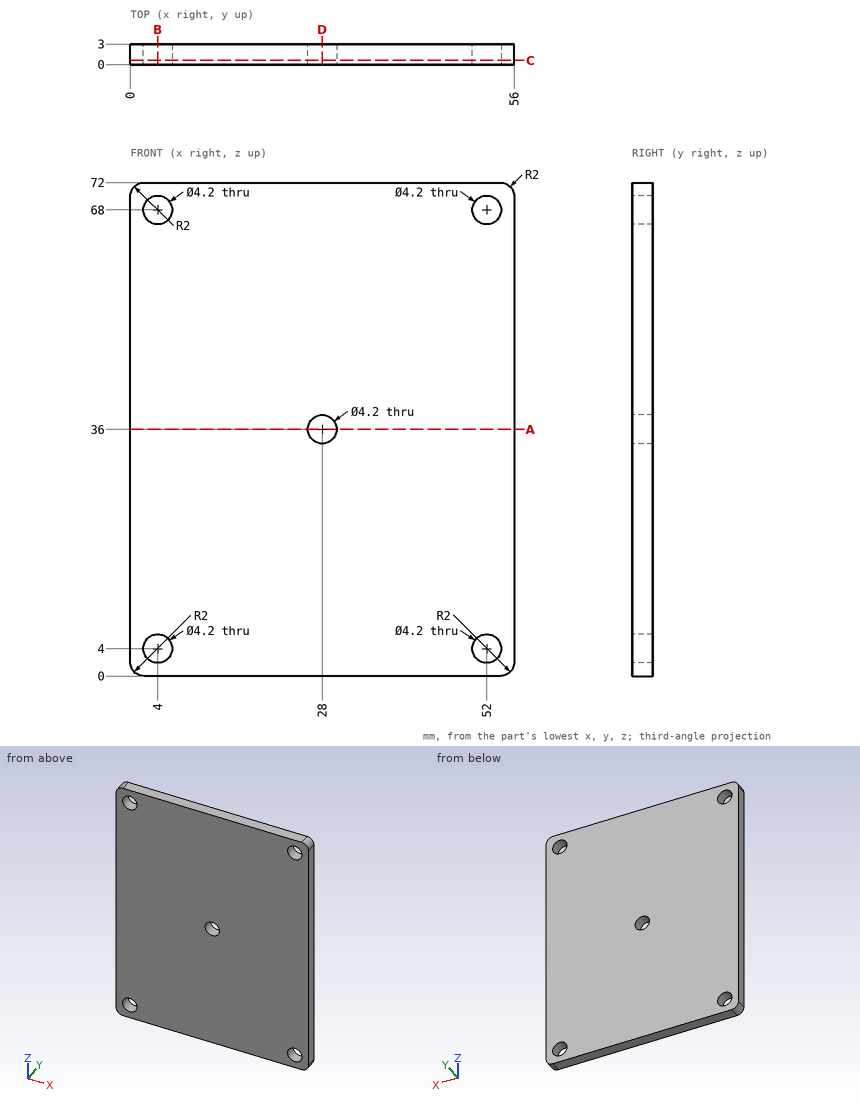
Drawing for the job (mm, zero at the part's lowest x, y, z). Round coordinates to 2 decimals unless told otherwise and drop trailing zeros. Write each loop counter-clockwise with the first axis right and the second up, starting at its lowest first coordinate (ties: lowest second). Pieces come first, ordered by that corner, then holes. Notation, with made-up numbers: (77.5, 45.25) - (112.5, 45.25) arc R35 cw to (112.5, 83.25) - close; hole circle Ø5 at (-11.5, 78). An arc over 180 degrees is marked (long way). Return JSON: item names as keys, results as strings. Group by question number.
Item 1: Band-saw the part on C-C on y = 0.6. List the corners of the cut face in (x, z), plus the area to 3 significant figures.
Item 2: Band-saw the part on A-A on z = 36. List the corners of the cut face in (x, y), plus the area to 3 significant figures.
Item 3: Band-saw the part on D-D on x = 28. List the corners of the cut face in (y, z), plus the area to 3 significant figures.
Item 4: Band-saw the part on B-B on x = 4. List the corners of the cut face in (y, z), plus the area to 3 significant figures.
Item 5: Probe probe 1 along Z at (x, y) = (4, 0.75). List the from-to ranges inside material, lowest first.
Resolved:
{
 "1": {"outline": "(0, 2) arc R2 ccw to (2, 0) - (54, 0) arc R2 ccw to (56, 2) - (56, 70) arc R2 ccw to (54, 72) - (2, 72) arc R2 ccw to (0, 70) - close; hole circle Ø4.2 at (4, 4); hole circle Ø4.2 at (4, 68); hole circle Ø4.2 at (28, 36); hole circle Ø4.2 at (52, 4); hole circle Ø4.2 at (52, 68)", "area": "3,960 mm²"},
 "2": {"outline": "(0, 0) - (25.9, 0) - (25.9, 3) - (0, 3) - close; (30.1, 0) - (56, 0) - (56, 3) - (30.1, 3) - close", "area": "155 mm²"},
 "3": {"outline": "(0, 0) - (3, 0) - (3, 33.9) - (0, 33.9) - close; (0, 38.1) - (3, 38.1) - (3, 72) - (0, 72) - close", "area": "203 mm²"},
 "4": {"outline": "(0, 0) - (3, 0) - (3, 1.9) - (0, 1.9) - close; (0, 6.1) - (3, 6.1) - (3, 65.9) - (0, 65.9) - close; (0, 70.1) - (3, 70.1) - (3, 72) - (0, 72) - close", "area": "191 mm²"},
 "5": {"probe 1": "z = 0 to 1.9, 6.1 to 65.9, 70.1 to 72"}
}
